from build123d import *

# Parameters (mm, degrees)
F0_R     = 3
F0_R_2   = 2.5
F1_DEPTH = 3
F2_DEPTH = 5


# Not quite as in the source:
# - ends of sketch curves that miss each other by under 0.0002 mm in the source are joined


with BuildPart() as f1:
    # F0 (on Top) → F1 (new body)
    with BuildSketch(Plane.XY):
        with BuildLine():
            Line((-1.7219635134, -9.6237825349), (-1.7162322612, -9.6237825349))
            Line((-1.7162322612, -9.6237825349), (2.1097812593, -9.6237806245))
            ThreePointArc((2.1097812593, -9.6237806245), (3.109244006, -9.5259463757), (4.0703036603, -9.2346361811))
            ThreePointArc((4.0703036603, -9.2346361811), (4.9367767363, -8.7689594925), (5.6928675676, -8.1397082139))
            ThreePointArc((5.6928675676, -8.1397082139), (6.3014355553, -7.384861889), (6.7518423579, -6.5262108466))
            ThreePointArc((6.7518423579, -6.5262108466), (7.0313366054, -5.5856490766), (7.1251796223, -4.6089367858))
            Line((7.1251796223, -4.6089367858), (7.1251795967, 0.4059089633))
            Line((7.1251795967, 0.4059089633), (3.3043447402, 0.4059089633))
            Line((3.3043447402, 0.4059089633), (3.3043447402, 9.6236730545))
            Line((3.3043447402, 9.6236730545), (-1.7092449094, 9.6236835618))
            ThreePointArc((-1.7092449094, 9.6236835618), (-2.0928177445, 9.6100571875), (-2.4738865464, 9.5642275806))
            ThreePointArc((-2.4738865464, 9.5642275806), (-2.8609393666, 9.4846946207), (-3.2402037336, 9.3738166285))
            ThreePointArc((-3.2402037336, 9.3738166285), (-3.6975405848, 9.1984368029), (-4.1390265018, 8.9862923546))
            ThreePointArc((-4.1390265018, 8.9862923546), (-4.5162413892, 8.7629757089), (-4.8714990411, 8.5061617901))
            ThreePointArc((-4.8714990411, 8.5061617901), (-5.2720148148, 8.1490003263), (-5.6296128286, 7.7488742742))
            ThreePointArc((-5.6296128286, 7.7488742742), (-5.9394367718, 7.3112544614), (-6.197789407, 6.8414078072))
            ThreePointArc((-6.197789407, 6.8414078072), (-6.3173685837, 6.5707517714), (-6.4204719372, 6.2934007888))
            ThreePointArc((-6.4204719372, 6.2934007888), (-6.5129249786, 5.9920188156), (-6.5882375678, 5.6859033621))
            ThreePointArc((-6.5882375678, 5.6859033621), (-6.6481890942, 5.3652316519), (-6.6899638063, 5.0416896752))
            ThreePointArc((-6.6899638063, 5.0416896752), (-6.7168439977, 4.6824291061), (-6.7253469337, 4.3222646908))
            Line((-6.7253469337, 4.3222646908), (-6.7253324298, -4.6083307059))
            ThreePointArc((-6.7253324298, -4.6083307059), (-6.6405112105, -5.5189445936), (-6.3874853783, -6.3978019019))
            ThreePointArc((-6.3874853783, -6.3978019019), (-5.9650696712, -7.2398337428), (-5.3973270448, -7.9915790132))
            ThreePointArc((-5.3973270448, -7.9915790132), (-5.0455065065, -8.3419922854), (-4.6606937322, -8.6558175446))
            ThreePointArc((-4.6606937322, -8.6558175446), (-4.2509916029, -8.9267871137), (-3.8162055499, -9.1553509281))
            ThreePointArc((-3.8162055499, -9.1553509281), (-3.3266240966, -9.3511061983), (-2.8189514749, -9.4935092865))
            ThreePointArc((-2.8189514749, -9.4935092865), (-2.2737789347, -9.586614675), (-1.7219635134, -9.6237825349))
        make_face()
        with Locations((0.1967744991, -4.6086336082)):
            Circle(F0_R, mode=Mode.SUBTRACT)
        with Locations((-1.6951942668, 4.3222646911)):
            Circle(F0_R_2, mode=Mode.SUBTRACT)
    extrude(amount=-F1_DEPTH)

    # F2 (add): a face of the model
    f2_faces = [f1.faces().sort_by_distance(p)[0] for p in [
        (7.1251796095, -2.1015139113, -1.5),
    ]]
    extrude(f2_faces, amount=F2_DEPTH)


solid = f1.part
Design review of the part built by this model. Coordinates are the model's own, in mm. A direction names the side the tool comes from. Coordinates: 2 decimals unless noted, no trailing zeros. Write each loop counter-clockwise with the first axis right and the second up, starting at its lowest first coordinate (ties: lowest second). Pieces come first, ordered by that corner, then holes. Notation, with made-up numbers: (29, 8) - (88, 8) arc R18 ccw to (88, 43) - close; hole circle Ø6 at (83.5, 59.5). An arc over 180 degrees is marked (long way). Use one line per item in the form item = value.
Q1. The part is to be moulded in two halves that separate along X. For faces 3 (the cylindrical face through (7.03, -5.6, -1.48)), 4 (the cylindrical face through (-2.281, -9.586, -1.479)), 5 (the cylindrical face through (-3.68, 2.8, -1.48)), say which applies: +X half, -X half, draft (parallel to the pull), parting line (faces both ways), or undercut.
Taken from the geometry:
face_3 = +X half
face_4 = -X half
face_5 = undercut
Q2. Machinability: for faces 1 (the flat face through (3.304, 5, -1)), 2 (the cylindrical face through (-5.935, 7.318, -1.479)), which of the approach directions +Z, -Z, +X, -X, +Y, -Y give a long, thin tool a straight path to every point of the face, cutting with its end or side? Answer none if there is none.
Taken from the geometry:
face_1 = +Z, -Z, +X, +Y
face_2 = +Z, -Z, -X, +Y
Q3. Consider section C-C (z = -0.6). Count the separate pieces of the cut face and the enclosed holes in it, plus the area to 3 significant figures.
Taken from the geometry:
separate_pieces = 1
enclosed_holes = 2
area = 192 mm^2
Q4. Consider section A-A (y = 2.25). Write out the cut boundary in (x, z).
Taken from the geometry:
outline = (-6.73, -3) - (-3.09, -3) - (-3.09, 0) - (-6.73, 0) - close; (-0.3, -3) - (3.3, -3) - (3.3, 0) - (-0.3, 0) - close
Q5. Consider section B-B (x = 0). Write out the cut boundary in (y, z), plus the area to 3 significant figures.
Taken from the geometry:
outline = (-9.62, -3) - (-7.6, -3) - (-7.6, 0) - (-9.62, 0) - close; (-1.62, -3) - (2.48, -3) - (2.48, 0) - (-1.62, 0) - close; (6.16, -3) - (9.62, -3) - (9.62, 0) - (6.16, 0) - close
area = 28.8 mm^2
Q6. For probe 1 along Y at (x, z) = (7.5, -0.55); probe 2 along X at (y, z) = (1, -0.3); probe 3 along X at (y, z) = (5.5, -1.55), list the stretches that pass through material, from the lowest coordinate up.
Taken from the geometry:
probe_1 = -4.61 to 0.41
probe_2 = -6.73 to 3.3
probe_3 = -6.63 to -3.9, 0.51 to 3.3
Q7. Consider section D-D (x = 2.75). Write out the cut boundary in (y, z).
Taken from the geometry:
outline = (-9.58, -3) - (-6.18, -3) - (-6.18, 0) - (-9.58, 0) - close; (-3.03, -3) - (9.62, -3) - (9.62, 0) - (-3.03, 0) - close
Q8. Insertion check: pin 1 Ø1 at (x, z) = (5.5, -0.5) entering from -Y; pin 2 Ø0.9 at (y, z) = (6, -1) entering from +X. Each pin has a flat end and moves straight along its axis. Give the tip position at first contact, or say it passes through.
Taken from the geometry:
pin_1 = -8.73
pin_2 = 3.3
